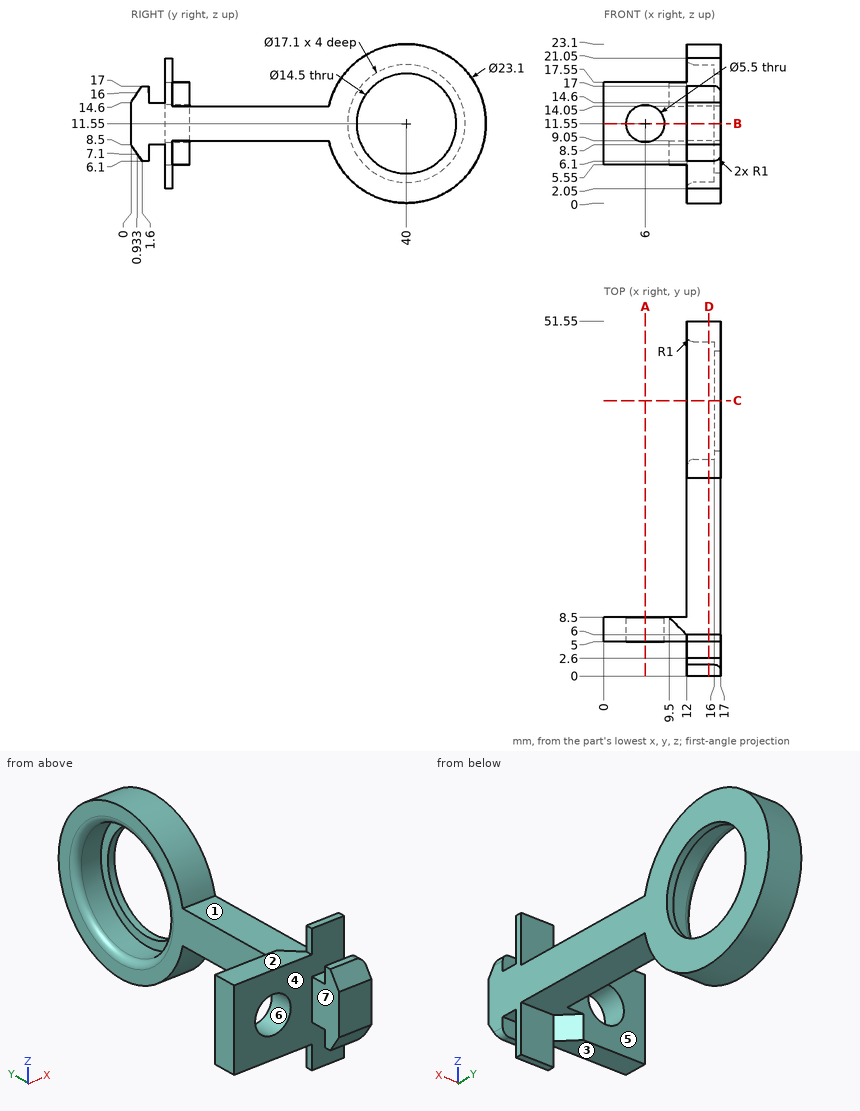
For this review, use the dimensioned drawing (mm, ordinates from the lowest corner) and the shaded views. A direction names the side the tool comes from. Round coordinates to 2 decimals unless told otherwise and drop trailing zeros. Write each loop counter-clockwise with the first axis right and the second up, starting at its lowest first coordinate (ties: lowest second). Pieces come first, ordered by that corner, then holes. Notation, with made-up numbers: (64.5, 42) - (114.5, 42) arc R20 cw to (114.5, 72) - close; hole circle Ø5 at (-14, 45). An arc over 180 degrees is marked (long way). Answer as a JSON object with one key per item and string values.
1. We need section A-A on x = 6. Give the boundary of the cut face in (y, z).
Response values:
{"outline": "(5, 5.55) - (8.5, 5.55) - (8.5, 8.8) - (5, 8.8) - close; (5, 14.3) - (8.5, 14.3) - (8.5, 17.55) - (5, 17.55) - close"}
2. We need section D-D on x = 15.25. Give the boundary of the cut face in (y, z).
Response values:
{"outline": "(0, 8.5) - (1.6, 6.1) - (2.6, 6.1) - (2.6, 8.5) - (5, 8.5) - (5, 2.05) - (6, 2.05) - (6, 9.05) - (28.72, 9.05) arc R11.55 ccw (long way) to (28.72, 14.05) - (6, 14.05) - (6, 21.05) - (5, 21.05) - (5, 14.6) - (2.6, 14.6) - (2.6, 17) - (1.6, 17) - (0, 14.6) - close; hole circle Ø17.1 at (40, 11.55)"}
3. Draft analysis for pull direction X (two halves, no side actions). For the marked faces 5, 6 and 7, state which applies: +X half, -X half, draft (parallel to the pull), parting line (faces both ways), or undercut.
Response values:
{"face 5": "draft", "face 6": "undercut", "face 7": "-X half"}
4. We need section B-B on z = 11.55. Give the boundary of the cut face in (x, y), then the cut area to 3 significant figures.
Response values:
{"outline": "(0, 5) - (3.25, 5) - (3.25, 8.5) - (0, 8.5) - close; (8.75, 5) - (12, 5) - (12, 0) - (17, 0) - (17, 32.75) - (16, 32.75) - (16, 31.45) - (13, 31.45) arc R1 ccw to (12, 30.45) - (12, 8.5) - (8.75, 8.5) - close; (12, 49.55) arc R1 ccw to (13, 48.55) - (16, 48.55) - (16, 47.25) - (17, 47.25) - (17, 51.55) - (12, 51.55) - close", "area": "197 mm2"}
5. Tool access review of the marked faces 1, 2, 3 and 4: name each direction out of +Z, -Z, +X, -X, +Y, -Y from which nothing blocks a thin tool from reaching the whole face with its end or side.
Response values:
{"face 1": "+Z, +X", "face 2": "+Z, -X, +Y, -Y", "face 3": "-Z, -X, +Y, -Y", "face 4": "-X"}
6. For pin 1 Ø2.5 at (x, z) = (15.5, 6.5) entering from +Y; pin 2 Ø1.5 at (x, z) = (6.5, 17.5) entering from +Y; pin 3 Ø1.5 at (x, z) = (13.5, 16.5) entering from +Y; pin 4 Ø2 at (x, y) = (10.5, 30.5) entering from +Z, all flat-tipped, find the tip position at first contact; note any pin that passes through.
Response values:
{"pin 1": "stops at y = 50.91", "pin 2": "stops at y = 8.5", "pin 3": "stops at y = 50.76", "pin 4": "passes through"}
7. To check wall thickness, follow line 1 along X through (y, z) = (7.85, 11.55); line 2 along Y through (x, z) = (16.8, 11.55); line 3 along Y through (x, z) = (12.75, 15.75) (1 decimal). State the ranges of each line that lie inside material, in increasing order.
Response values:
{"line 1": "x = 0 to 3.25, 8.75 to 17", "line 2": "y = 0 to 32.75, 47.25 to 51.55", "line 3": "y = 0.8 to 2.6, 5 to 6, 29.2 to 32.5, 47.5 to 50.8"}
8. We need section C-C on y = 40. Give the boundary of the cut face in (x, z).
Response values:
{"outline": "(12, 0) - (17, 0) - (17, 4.3) - (16, 4.3) - (16, 3) - (13, 3) arc R1 ccw to (12, 2) - close; (12, 21.1) arc R1 ccw to (13, 20.1) - (16, 20.1) - (16, 18.8) - (17, 18.8) - (17, 23.1) - (12, 23.1) - close"}
